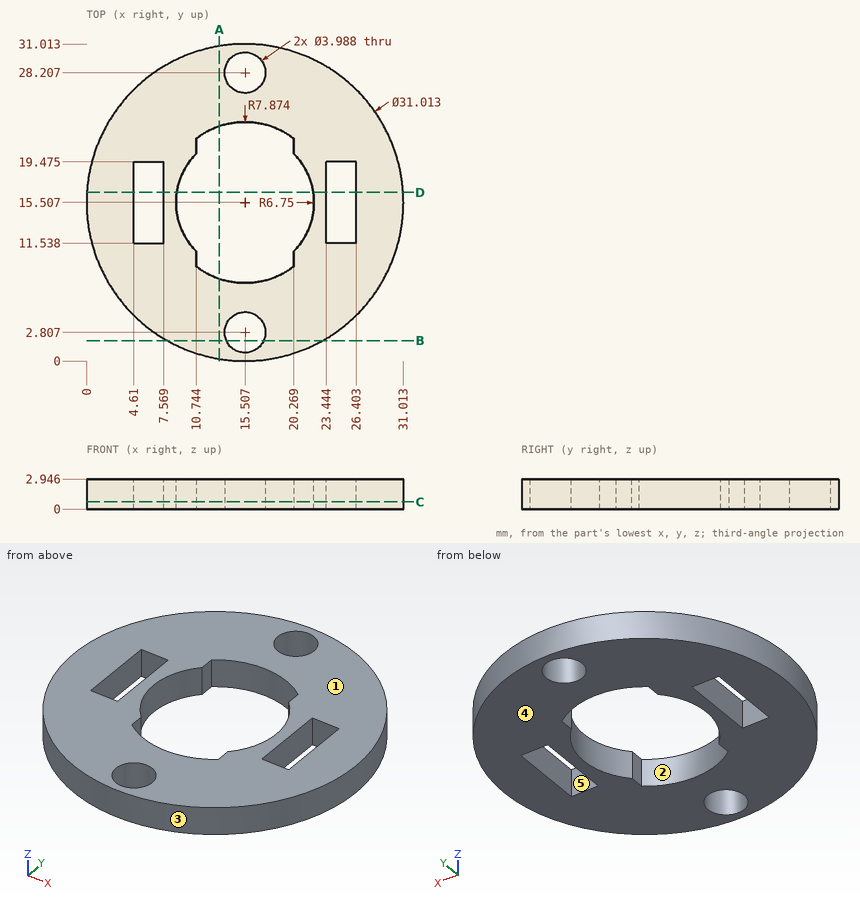
Input: dimensioned drawing with shaded views. Units: mm. Origin: part minimum x, y, z. A direction names the side the tool comes from. Coordinates: 2 decimals unless noted, no trailing zeros. Order: outer loops, then holes, each group sorted by start corner. A loop starts at its lowest first (then second) coordinate and runs counter-clockwise, first axis right, second up. Notation, with made-up numbers: M 80,34.25 L 128,34.25 A23 ccw 128,61.25 Z; hole C 66.25,-40 d11. An arc over 180 degrees is marked long. Answer as CSV lines item,"result".
Q1. First-contact query: P1, Ø1.5, axis at x = 6, z = 2, coming from the -Y side; P2, Ø1.5, axis at x = 25, z = 1.5, coming from the +Y side; P3, Ø0.9, axis at x = 25.5, z = 2, coming from the -Y side (1 decimal). Flat tips, straight axial feed; report the tip coordinate or a pass-through.
Answers:
P1,"stops at y = 2.71"
P2,"stops at y = 28.31"
P3,"stops at y = 3.3"
Q2. Line query: probe 1 along Y at (x, z) = (16, 0.8) (1 decimal); probe 2 along X at (y, z) = (12, 0.4) (1 decimal); probe 3 along Y at (x, z) = (13, 1.55) (1 decimal). Output: solid intervals per line, ascending. Write a range as [from, to].
Answers:
probe 1,"y = [0, 0.9], [4.7, 7.6], [23.4, 26.3], [30.1, 31]"
probe 2,"x = [0.4, 4.6], [7.6, 9.7], [21.3, 23.4], [26.4, 30.6]"
probe 3,"y = [0.2, 8], [23, 30.8]"
Q3. Draft query along X for the marked faces 1, 2 and 3. Return one class per face: pulls with the +X half, pulls with the -X half, needs draft (parallel to the pull), parting line crosses it, or undercut.
Answers:
face 1,"needs draft"
face 2,"undercut"
face 3,"parting line crosses it"
Q4. Section D-D on y = 16.5. Return the cut outline in (x, z) (1 decimal).
Answers:
outline,"M 0,0 L 4.6,0 L 4.6,2.9 L 0,2.9 Z; M 7.6,0 L 8.8,0 L 8.8,2.9 L 7.6,2.9 Z; M 22.2,0 L 23.4,0 L 23.4,2.9 L 22.2,2.9 Z; M 26.4,0 L 31,0 L 31,2.9 L 26.4,2.9 Z"
Q5. Section C-C on z = 0.7. Count the separate pieces of the cut face and the enclosed holes in it, and give its area (3 significant figures).
Answers:
separate pieces,"1"
enclosed holes,"5"
area,"517 mm^2"
Q6. Section B-B on y = 2. Return the cut outline in (x, z) (1 decimal).
Answers:
outline,"M 7.9,0 L 13.7,0 L 13.7,2.9 L 7.9,2.9 Z; M 17.3,0 L 23.1,0 L 23.1,2.9 L 17.3,2.9 Z"
Q7. Set-up query: the marked faces 4 and 5. Return all of +Z, -Z, +X, -X, +Y, -Y with unobstructed straight access to the full face (end or side cutting, diameter ignored); none if empty.
Answers:
face 4,"-Z, +X, -X, +Y, -Y"
face 5,"+Z, -Z"
Q8. Section A-A on x = 13. Return the cut outline in (y, z), and give its area (3 significant figures).
Answers:
outline,"M 0.2,0 L 8.04,0 L 8.04,2.95 L 0.2,2.95 Z; M 22.97,0 L 30.81,0 L 30.81,2.95 L 22.97,2.95 Z"
area,"46.2 mm^2"
